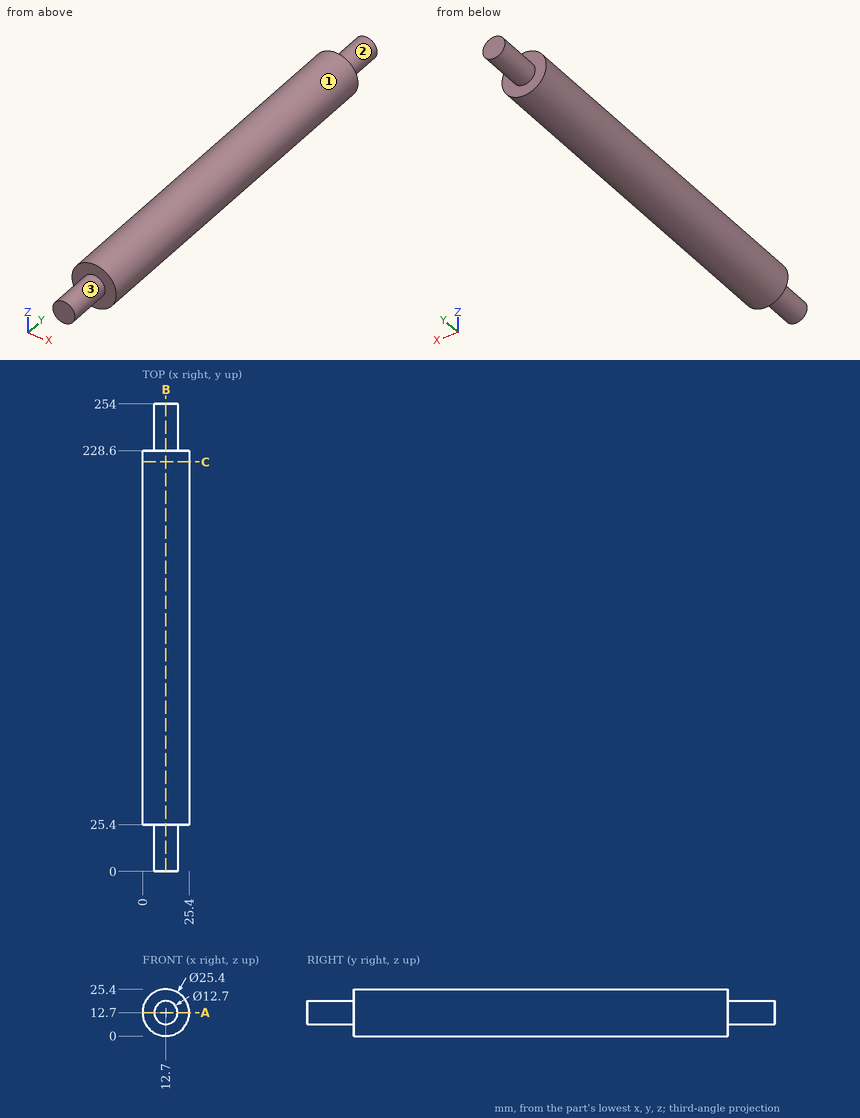
Geometry: see drawing. Coordinates: mm, zero at the bounding-box minimum. A direction names the side the tool comes from. Coordinates: 2 decimals unless noted, no trailing zeros. Loops run counter-clockwise (first coordinate to the right, second up) from the corner with the lowest first, then second, coordinate; pieces in that order, holes last. Notation, with made-up numbers: (45.5, 52) -> (93.5, 52) arc R3 cw to (93.5, 56) -> close; hole circle Ø8 at (-28.5, 77.25). An arc over 180 degrees is marked (long way). Use a Markdown table: item, result.
1) Contact query for flat-ended pins moving along their axis: pin 1 (12 mm diameter, centred on x = 3, y = 130.5, fed in from +Z); pin 2 (3 mm diameter, centred on x = 19.5, z = 4, fed in from +Y); pin 3 (1.5 mm diameter, centred on y = 216.5, z = 14, fed in from +X). Output: stop coordinate, or through.
Results found:
| item | result |
|---|---|
| pin 1 | stops at z = 24.85 |
| pin 2 | stops at y = 228.6 |
| pin 3 | stops at x = 25.39 |
2) Cut plane C-C (y = 222.5). Return the cut outline in (x, z), then the cut area to 3 significant figures.
Results found:
| item | result |
|---|---|
| outline | circle Ø25.4 at (12.7, 12.7) |
| area | 507 mm2 |
3) Access query for the marked faces 1, 2 and 3. Directions: +Z, -Z, +X, -X, +Y, -Y. A direction counts if a zero-diameter tool reaches every point of the face in a straight line with its end or side. Return the directions, or none.
Results found:
| item | result |
|---|---|
| face 1 | +Y, -Y |
| face 2 | +Y |
| face 3 | -Y |
4) Cut plane A-A (z = 12.7). Return the cut outline in (x, y), then the cut area to 3 significant figures.
Results found:
| item | result |
|---|---|
| outline | (0, 25.4) -> (6.35, 25.4) -> (6.35, 0) -> (19.05, 0) -> (19.05, 25.4) -> (25.4, 25.4) -> (25.4, 228.6) -> (19.05, 228.6) -> (19.05, 254) -> (6.35, 254) -> (6.35, 228.6) -> (0, 228.6) -> close |
| area | 5,810 mm2 |
5) Cut plane B-B (x = 12.7). Return the cut outline in (y, z), then the cut area to 3 significant figures.
Results found:
| item | result |
|---|---|
| outline | (0, 6.35) -> (25.4, 6.35) -> (25.4, 0) -> (228.6, 0) -> (228.6, 6.35) -> (254, 6.35) -> (254, 19.05) -> (228.6, 19.05) -> (228.6, 25.4) -> (25.4, 25.4) -> (25.4, 19.05) -> (0, 19.05) -> close |
| area | 5,810 mm2 |
6) Material intervals for line 1 along Y through (x, z) = (6.5, 20.25); line 2 along Z through (x, y) = (11.75, 184); line 3 along Z through (x, y) = (6.75, 144), sorted ascending. Write a range as from..to.
Results found:
| item | result |
|---|---|
| line 1 | y = 25.4..228.6 |
| line 2 | z = 0.04..25.36 |
| line 3 | z = 1.48..23.92 |
